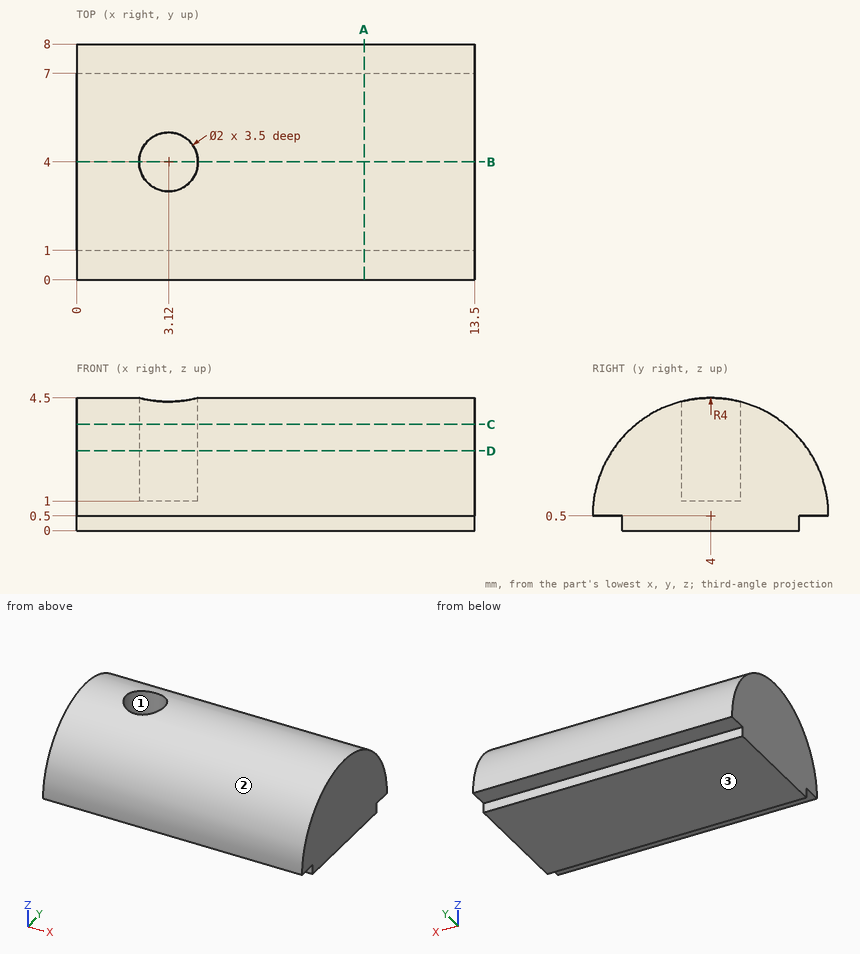
The figure shows three views and two pictorial views of one solid part (mm, origin at its lowest corner). Answer the questions. Give positions to 0.01 mm unless a question says otherwise; leave off trailing zeros. Write each loop counter-clockwise with the first axis right and the second up, starting at its lowest first coordinate (ties: lowest second). Pieces come first, ordered by that corner, then holes. Notation, with made-up numbers: M 63.5,-30.75 L 67.5,-30.75 A23 ccw 67.5,-3.75 Z; hole C 59.25,20 d3. An arc over 180 degrees is marked long. One line per item, written item: value. Start each with the question number.
(1) Find section D-D (z = 2.7). Determine the outline of the cut face in (x, y).
(2) Find section C-C (z = 3.6). Determine the outline of the cut face in (x, y).
(3) Find section A-A (x = 9.75). Determine the outline of the cut face in (y, z).
(4) Find section B-B (y = 4). Determine the outline of the cut face in (x, z), plus the area to 4 significant figures.
(5) Find the intervals of material crossed by line 1 (Y direction, x = 3.12, z = 3.35); line 2 (Y direction, x = 3.12, z = 3.05); line 3 (Z direction, x = 2.75, y = 4), in increasing order.
(6) Determine the mould class of the marked faces 1, 2 and 3 for opening direction Y: pulls with the +Y half, pulls with the -Y half, needs draft (parallel to the pull), parting line crosses it, or undercut.
(7) Flat-ended cylindrical pins translate along their axes: pin 1 Ø2 at (x, z) = (4, 3.5) entering from -Y; pin 2 Ø4 at (x, y) = (7.5, 5.5) entering from +Z; pin 3 Ø4 at (x, y) = (6, 1) entering from +Z; pin 4 Ø1 at (x, y) = (3.5, 4) entering from +Z. Find the tip coordinate at first contact, or state that the pin passes through.
Results below:
1. outline: M 0,0.66 L 13.5,0.66 L 13.5,7.34 L 0,7.34 Z; hole C 3.12,4 d2
2. outline: M 0,1.47 L 13.5,1.47 L 13.5,6.53 L 0,6.53 Z; hole C 3.12,4 d2
3. outline: M 0,0.5 L 1,0.5 L 1,0 L 7,0 L 7,0.5 L 8,0.5 A4 ccw Z
4. outline: M 0,0 L 13.5,0 L 13.5,4.5 L 4.12,4.5 L 4.12,1 L 2.12,1 L 2.12,4.5 L 0,4.5 Z
4. area: 53.75 mm^2
5. line 1: y = 1.19 to 3, 5 to 6.81
5. line 2: y = 0.92 to 3, 5 to 7.08
5. line 3: z = 0 to 1
6. face 1: undercut
6. face 2: parting line crosses it
6. face 3: needs draft
7. pin 1: stops at y = 0.54
7. pin 2: stops at z = 4.5
7. pin 3: stops at z = 4.37
7. pin 4: stops at z = 1
